Drawing for the job (mm, zero at the part's lowest x, y, z). Round coordinates to 2 decimals unless told otherwise and drop trailing zeros. Write each loop counter-clockwise with the first axis right and the second up, starting at its lowest first coordinate (ties: lowest second). Pieces come first, ordered by that corner, then holes. Notation, with made-up numbers: (42.5, 11.5) -> (78.5, 11.5) arc R8 ccw to (78.5, 24.5) -> close; hole circle Ø1 at (64, 64.5). An arc over 180 degrees is marked (long way). One line per question, with ' | ' between items.
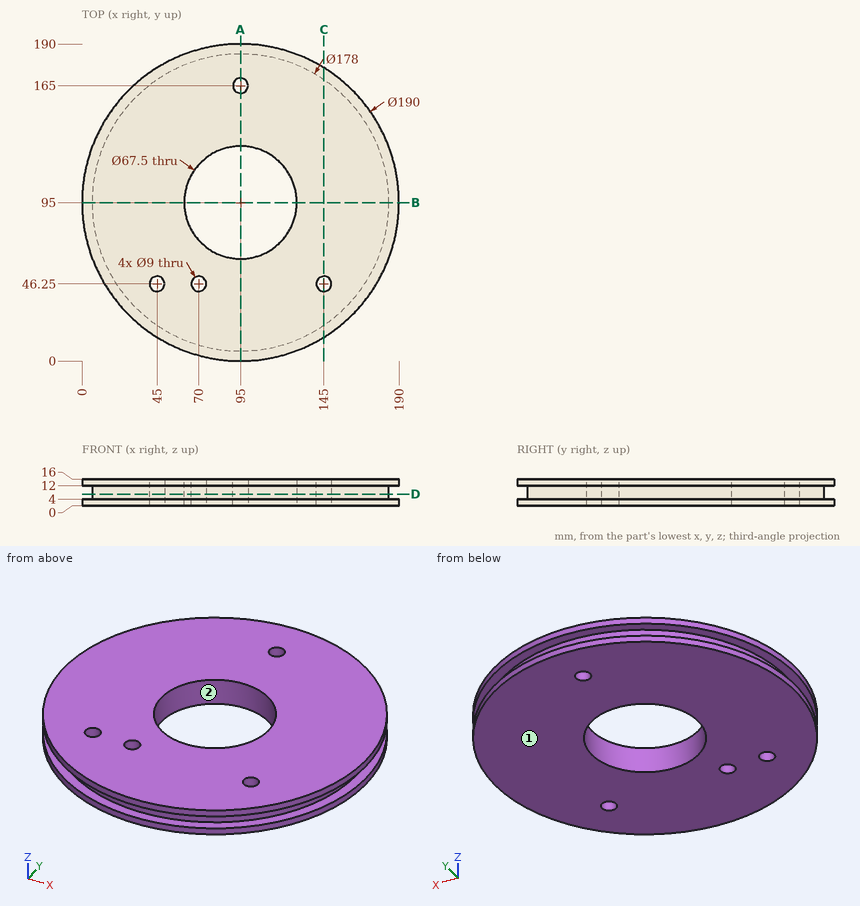
(1) Wall check: line 1 (Y direction, x = 95, z = 5); line 2 (Z direction, x = 145.5, y = 17); line 3 (Y direction, x = 97.5, z = 7.5). Give the ranges that are in metal, low to high. Write a range as from..to.
Calculated:
line 1: 6..61.25, 128.75..160.5, 169.5..184 | line 2: 0..4, 12..16 | line 3: 6.04..61.34, 128.66..161.26, 168.74..183.96
(2) Slice it at B-B (y = 95). Write the cut outline in (x, z).
Calculated:
outline: (0, 0) -> (61.25, 0) -> (61.25, 16) -> (0, 16) -> (0, 12) -> (6, 12) -> (6, 4) -> (0, 4) -> close; (128.75, 0) -> (190, 0) -> (190, 4) -> (184, 4) -> (184, 12) -> (190, 12) -> (190, 16) -> (128.75, 16) -> close
(3) Slice it at D-D (z = 7). Write the cut outline in (x, y), then the cut area to 3 significant figures.
Calculated:
outline: circle Ø178 at (95, 95); hole circle Ø9 at (45, 46.25); hole circle Ø67.5 at (95, 95); hole circle Ø9 at (70, 46.25); hole circle Ø9 at (95, 165); hole circle Ø9 at (145, 46.25) | area: 21,100 mm2
(4) Slice it at C-C (x = 145). Write the cut outline in (y, z).
Calculated:
outline: (14.22, 0) -> (41.75, 0) -> (41.75, 16) -> (14.22, 16) -> (14.22, 12) -> (21.37, 12) -> (21.37, 4) -> (14.22, 4) -> close; (50.75, 0) -> (175.78, 0) -> (175.78, 4) -> (168.63, 4) -> (168.63, 12) -> (175.78, 12) -> (175.78, 16) -> (50.75, 16) -> close
(5) Mould opens along X. For the marked faces 1 and 2 say: pulls with the +X half, pulls with the -X half, needs draft (parallel to the pull), parting line crosses it, or undercut.
Calculated:
face 1: needs draft | face 2: undercut
(6) Drop flat-ended pins along their axis: pin 1 (2 mm diameter, centred on y = 110.5, z = 6, fed in from +X); pin 2 (4 mm diameter, centred on x = 71.5, z = 12, fed in from -Y); pin 3 (8 mm diameter, centred on x = 95, y = 165, fed in from -Z); pin 4 (3 mm diameter, centred on y = 39, z = 12, fed in from -X). Give the stop position or say it passes through.
Calculated:
pin 1: x = 182.81 | pin 2: y = 2.46 | pin 3: through | pin 4: x = 17.19
(7) Slice it at A-A (x = 95). Write the cut outline in (y, z).
Calculated:
outline: (0, 0) -> (61.25, 0) -> (61.25, 16) -> (0, 16) -> (0, 12) -> (6, 12) -> (6, 4) -> (0, 4) -> close; (128.75, 0) -> (160.5, 0) -> (160.5, 16) -> (128.75, 16) -> close; (169.5, 0) -> (190, 0) -> (190, 4) -> (184, 4) -> (184, 12) -> (190, 12) -> (190, 16) -> (169.5, 16) -> close
